from build123d import *

# Parameters (mm, degrees)
F0_R     = 3
F0_R_2   = 2.5
F1_DEPTH = 17.5
F3_W     = 6
F3_H     = 6
F4_DEPTH = 0.5
F6_R     = 2
F7_R     = 1
F5_R     = 1.75
F8_DEPTH = 25


with BuildPart() as f1:
    # F0 (on Right) → F1 (new body, symmetric)
    with BuildSketch(Plane.YZ):
        Circle(F0_R)
        Circle(F0_R_2, mode=Mode.SUBTRACT)
    extrude(amount=F1_DEPTH, both=True)

    # F3 (on offset) → F4 (join)
    with BuildSketch(Plane.XY.offset(-3)):
        with Locations((20.5, 0)):
            Rectangle(F3_W, F3_H)
        with Locations((-20.5, 0)):
            Rectangle(F3_W, F3_H)
    extrude(amount=F4_DEPTH)

    # F6
    f6_edges = [f1.edges().sort_by_distance(p)[0] for p in [
        (23.5, 3, -2.75),
        (23.5, -3, -2.75),
        (-23.5, -3, -2.75),
        (-23.5, 3, -2.75),
    ]]
    fillet(f6_edges, radius=F6_R)

    # F7
    f7_edges = [f1.edges().sort_by_distance(p)[0] for p in [
        (17.5, -3, -2.75),
        (17.5, 3, -2.75),
        (-17.5, -3, -2.75),
        (-17.5, 3, -2.75),
    ]]
    fillet(f7_edges, radius=F7_R)

    # F5 (on face) → F8 (cut)
    with BuildSketch(Plane.XY.offset(-2.5)):
        with Locations((20, 0)):
            Circle(F5_R)
        with Locations((-20, 0)):
            Circle(F5_R)
    extrude(amount=-F8_DEPTH, mode=Mode.SUBTRACT)


solid = f1.part
Here's how the part is built. I have some questions about the finished solid (model axes, mm). A direction names the side the tool comes from. Coordinates: 2 decimals unless noted, no trailing zeros. Order: outer loops, then holes, each group sorted by start corner. A loop starts at its lowest first (then second) coordinate and runs counter-clockwise, first axis right, second up.
Item 1: If we section it at C-C on x = -2: List the corners of the cut face in (y, z) for me, plus the area to 3 significant figures.
Result sheet:
outline: circle Ø6 at (0, 0); hole circle Ø5 at (0, 0)
area: 8.64 mm2
Item 2: If we mould it in two halves opening along X, with no side actions, what happens to faces 1 (the face through (-22.9, 2.43, -2.75)), 2 (the face through (22.93, 2.4, -2.75)), 3 (the face through (22, 0, -3)), 4 (the face through (0, -3, 0))? For each: +X half, -X half, draft (parallel to the pull), parting line (faces both ways), or undercut.
Result sheet:
face 1: -X half
face 2: +X half
face 3: draft
face 4: undercut
Item 3: If we section it at A-A on z = 0: List the corners of the cut face in (x, y) for me.
Result sheet:
outline: (-17.5, -3) - (17.5, -3) - (17.5, -2.5) - (-17.5, -2.5) - close; (-17.5, 2.5) - (17.5, 2.5) - (17.5, 3) - (-17.5, 3) - close
Item 4: If we section it at B-B on x = 20: List the corners of the cut face in (y, z) for me, plus the area to 3 significant figures.
Result sheet:
outline: (-3, -3) - (-1.75, -3) - (-1.75, -2.5) - (-3, -2.5) - close; (1.75, -3) - (3, -3) - (3, -2.5) - (1.75, -2.5) - close
area: 1.25 mm2
Item 5: For faces 5 (the face through (22.9, -2.43, -2.75)), 6 (the face through (22, 0, -2.5)), 7 (the face through (-22, 0, -2.5)), which set-ups out of +Z, -Z, +X, -X, +Y, -Y let a thin tool reach every point of the face, with its end or its side?
Result sheet:
face 5: +Z, -Z, +X, -Y
face 6: +Z, +X, +Y, -Y
face 7: +Z, -X, +Y, -Y
Item 6: I need wall thicknesses on line 1 (Y direction, x = 7.5, z = 0); line 2 (Y direction, x = 20, z = -2.7); line 3 (X direction, y = -1.5, z = 2.05). Which ranges of each line are inside material? Lowest first, please.
Result sheet:
line 1: y = -3 to -2.5, 2.5 to 3
line 2: y = -3 to -1.75, 1.75 to 3
line 3: x = -17.5 to 17.5
Item 7: For P1, Ø1, axis at x = -5.5, y = 2, coming from the -Z side; P2, Ø3, axis at x = 19.5, y = -0.5, coming from the +Z side, each with a flat end and sliding along its axis, tell me the tip position at first contact or that it passes through.
Result sheet:
P1: stops at z = -2.6
P2: stops at z = -2.5
